Verification items for the finished model (mm, model axes). A direction names the side the tool comes from. Round coordinates to 2 decimals unless told otherwise and drop trailing zeros. Write each loop counter-clockwise with the first axis right and the second up, starting at its lowest first coordinate (ties: lowest second). Pieces come first, ordered by that corner, then holes. Notation, with made-up numbers: M 35.25,9.25 L 40.25,9.25 A15 ccw 40.25,38.25 Z; hole C -18,49 d1. An arc over 180 degrees is marked long. Answer in a Markdown table with one row per item. Add a question column.
1. Go/stop test with flat-tipped pins: pin 1 Ø6 at (x, y) = (-5.5, 14.5) entering from -Z; pin 2 Ø13.5 at (x, z) = (-3, -0.5) entering from +Y; pin 3 Ø6 at (y, z) = (41, 9.5) entering from +X; pin 4 Ø1.5 at (x, z) = (-5, 9) entering from +Y. Record where each tip stops, or that it passes through.
2. Set-up check for faces 1 (the flat face through (0, 80, -8)), 2 (the cylindrical face through (10.835, 83.479, -8.308)), 3 (the flat face through (0, 85, -9)): record each of +Z, -Z, +X, -X, +Y, -Y from which the full face is reachable in a straight line by a thin tool's end or side.
3. Sectioned sample at A-A on y = 60.5. Record the cut outline in (x, z), plus the area to 3 significant figures.
4. Material ranges on probe 1 along Y at (x, z) = (-8, -4.25); probe 2 along Z at (x, y) = (-0.5, 75); probe 3 along Z at (x, y) = (-6, 54), recorded low to high.
```python
from build123d import *

# Parameters (mm, degrees)
F0_R      = 7.5
F1_DEPTH  = 80
F2_R      = 13.654
F3_DEPTH  = 5
F4_R      = 8.6540002376
F5_DEPTH  = 3
F5_FACE_R = 8.6540002376
F7_SIZE   = 2


# Not quite as in the source:
# - an extrude whose draft closes it to a point is written as a loft to that point


with BuildPart() as f1:
    # F0 (on Front) → F1 (new body)
    with BuildSketch(Plane.XZ):
        Circle(F0_R)
    extrude(amount=-F1_DEPTH)

    # F2 (on face) → F3 (join)
    with BuildSketch(Plane(origin=(0, 80, 0), x_dir=(-1, 0, 0), z_dir=(0, 1, 0))):
        Circle(F2_R)
    extrude(amount=F3_DEPTH)

    # F4 (on face) → F5 (join)
    with BuildSketch(Plane(origin=(0, 85, 0), x_dir=(-1, 0, 0), z_dir=(0, 1, 0))):
        Circle(F4_R)
    extrude(amount=F5_DEPTH)

    # F5_face (on face) → F6 section 0
    with BuildSketch(Plane(origin=(0, 88, 0), x_dir=(-1, 0, 0), z_dir=(0, 1, 0)), mode=Mode.PRIVATE) as f6_s0:
        Circle(F5_FACE_R)
    loft([f6_s0.sketch, Vertex(0, 111.7766702407, 0)], ruled=True)

    # F7
    f7_edges = [f1.edges().sort_by_distance(p)[0] for p in [
        (-7.5, 0, 0),
        (13.654, 80, 0),
    ]]
    chamfer(f7_edges, length=F7_SIZE)


solid = f1.part
```
Geometry check:
| question | item | result |
|---|---|---|
| 1 | pin 1 | stops at z = -7.07 |
| 1 | pin 2 | stops at y = 111.78 |
| 1 | pin 3 | stops at x = 3.74 |
| 1 | pin 4 | stops at y = 85 |
| 2 | face 1 | -Y |
| 2 | face 2 | +Y, -Y |
| 2 | face 3 | +Y |
| 3 | outline | C 0,0 d15 |
| 3 | area | 177 mm2 |
| 4 | probe 1 | y = 80 to 85 |
| 4 | probe 2 | z = -7.48 to 7.48 |
| 4 | probe 3 | z = -4.5 to 4.5 |
